Read the model definition and answer for the solid it produces. Units are mm, in the model's axes. A direction names the side the tool comes from. Coordinates: 2 decimals unless noted, no trailing zeros. Write each loop counter-clockwise with the first axis right and the second up, starting at its lowest first coordinate (ties: lowest second). Pieces come first, ordered by that corner, then holes. Notation, with made-up numbers: M 64.25,-9 L 95.25,-9 A25 ccw 95.25,7 Z; hole C -27.5,31.5 d10. An arc over 180 degrees is marked long. Write item = value, one per line.
from build123d import *

# Parameters (mm, degrees)
SKETCH010_R       = 2.5
SKETCH010_R_2     = 1.25
PAD008_DEPTH      = 15
BOX001_W          = 11
BOX001_H          = 10
BOX001_DEPTH      = 10
BOX002_W          = 10
BOX002_H          = 10
BOX002_DEPTH      = 10
CHAMFER002_SIZE   = 3
CYLINDER004_R     = 7
CYLINDER004_DEPTH = 3
CYLINDER005_R     = 4
CYLINDER005_DEPTH = 31


with BuildPart() as part:
    # Sketch010 → Pad008 (new body)
    with BuildSketch(Plane.XZ):
        with BuildLine():
            Line((0, 35), (5, 35))
            Line((5, 35), (5, 15))
            Line((5, 15), (0, 15))
            Line((0, 15), (0, 0))
            Line((0, 0), (12, 0))
            Line((12, 0), (12, 59.38))
            Line((12, 59.38), (7, 59.38))
            ThreePointArc((7, 59.38), (5.585786, 58.794214), (5, 57.38))
            Line((5, 57.38), (5, 43))
            Line((5, 43), (0, 43))
            ThreePointArc((0, 43), (-4, 39), (0, 35))
        make_face()
        with Locations((0, 39)):
            Circle(SKETCH010_R, mode=Mode.SUBTRACT)
        with Locations((8, 56.38)):
            Circle(SKETCH010_R_2, mode=Mode.SUBTRACT)
    extrude(amount=PAD008_DEPTH)

    # Box001 → Box001 (cut)
    with BuildSketch(Plane(origin=(-6.5, -2.5, 34), x_dir=(1, 0, 0), z_dir=(0, 0, 1))):
        with Locations((5.5, 5)):
            Rectangle(BOX001_W, BOX001_H)
    extrude(amount=BOX001_DEPTH, mode=Mode.SUBTRACT)

    # Box002 → Box002 (cut)
    with BuildSketch(Plane(origin=(-5.5, -21.5, 34), x_dir=(1, 0, 0), z_dir=(0, 0, 1))):
        with Locations((5, 5)):
            Rectangle(BOX002_W, BOX002_H)
    extrude(amount=BOX002_DEPTH, mode=Mode.SUBTRACT)

    # Chamfer002
    chamfer002_edges = [part.edges().sort_by_distance(p)[0] for p in [
        (0, -15, 7.5),
    ]]
    chamfer(chamfer002_edges, length=CHAMFER002_SIZE)

    # Cylinder004 → Cylinder004 (cut)
    with BuildSketch(Plane(origin=(8, -6, 56), x_dir=(1, 0, 0), z_dir=(0, -1, 0))):
        Circle(CYLINDER004_R)
    extrude(amount=CYLINDER004_DEPTH, mode=Mode.SUBTRACT)

    # Cylinder005 → Cylinder005 (cut)
    with BuildSketch(Plane(origin=(0, -7.5, 0), x_dir=(1, 0, 0), z_dir=(0, 0, 1))):
        Circle(CYLINDER005_R)
    extrude(amount=CYLINDER005_DEPTH, mode=Mode.SUBTRACT)


solid = part.part
Item 1: Find section B-B (y = -1.25). Determine the outline of the cut face in (x, z), and give its area (3 significant figures).
Worked answers:
outline = M 0,0 L 12,0 L 12,59.38 L 7,59.38 A2 ccw 5,57.38 L 5,43 L 4.5,43 L 4.5,35 L 5,35 L 5,15 L 0,15 Z; hole C 8,56.38 d2.5
area = 489 mm²
Item 2: Find section A-A (z = 53). Determine the outline of the cut face in (x, y), and give its area (3 significant figures).
Worked answers:
outline = M 5,-15 L 12,-15 L 12,-9 L 5,-9 Z; M 5,-6 L 12,-6 L 12,0 L 5,0 Z
area = 84.0 mm²
Item 3: For a pull along Y with two mould halves and no side action, classify faces 6 (the face through (8, -15, 30)), 7 (the face through (8.53, -7.48, 49.02)), 8 (the face through (10, -12, 59.38)) as released by +Y, released by -Y, zero draft, split by the parting line, or undercut.
Worked answers:
face_6 = released by -Y
face_7 = undercut
face_8 = zero draft
Item 4: Consider line 1 along X through (y, z) = (-3.6, 56.38); line 2 along Z through (x, y) = (8, -13.35); line 3 along X through (y, z) = (-9.5, 39). Determine where each line is inside the solid, lowest interval first. Write a range as from..to.
Worked answers:
line_1 = 5..6.75, 9.25..12
line_2 = 0..55.13, 57.63..59.38
line_3 = -4..-2.5, 2.5..12
Item 5: Find section C-C (x = 8). Determine the outline of the cut face in (y, z).
Worked answers:
outline = M -15,0 L 0,0 L 0,55.13 L -6,55.13 L -6,49 L -9,49 L -9,55.13 L -15,55.13 Z; M -15,57.63 L -9,57.63 L -9,59.38 L -15,59.38 Z; M -6,57.63 L 0,57.63 L 0,59.38 L -6,59.38 Z
Item 6: Which of the six approach directions +Z, -Z, +X, -X, +Y, -Y give full straight-line access (tool end or side, diameter ignored) to faces 1 (the face through (5, -7, 25)), 2 (the face through (3, -7, 43)), 3 (the face through (4.5, -1, 39)), 4 (the face through (2, -11.5, 41)), 5 (the face through (7.84, -2.96, 57.62))?
Worked answers:
face_1 = -X, +Y, -Y
face_2 = +Z, -X, +Y, -Y
face_3 = +Z, -X, +Y
face_4 = +Z, -X, -Y
face_5 = +Y, -Y
Item 7: Find section D-D (z = 12). Determine the outline of the cut face in (x, y).
Worked answers:
outline = M 0,-12 L 3,-15 L 12,-15 L 12,0 L 0,0 L 0,-3.5 A4 cw 0,-11.5 Z
Item 8: Flat-ended cylindrical pins translate along their axes: pin 1 (4 mm diameter, centred on x = 0, z = 40, fed in from -Y); pin 2 (4 mm diameter, centred on x = 2.5, y = -10, fed in from +Z); pin 3 (1 mm diameter, centred on y = -2, z = 5, fed in from -X). Find the tip coordinate at first contact, or state that the pin passes through.
Worked answers:
pin_1 = -11.5
pin_2 = 43
pin_3 = 0
